Check sheet for the modelled part. Datum: model origin and axes. Units: mm. Coordinates: 2 decimals unless noted, no trailing zeros. Order: outer loops, then holes, each group sorted by start corner. A loop starts at its lowest first (then second) coordinate and runs counter-clockwise, first axis right, second up.
from build123d import *

# Parameters (mm, degrees)
EXTRUDE_1_DEPTH = 6
FILLET_1_R      = 0.5


with BuildPart() as part:
    # 草图1 → 凸台-拉伸1 (new body)
    with BuildSketch(Plane.XY):
        with BuildLine():
            Line((-9.3, 0), (-9.3, -15.9))
            Line((-9.3, -15.9), (9.3, -15.9))
            Line((9.3, -15.9), (9.3, 0))
            ThreePointArc((9.3, 0), (0, 9.3), (-9.3, 0))
        make_face()
    extrude(amount=EXTRUDE_1_DEPTH)

    # 圆角1
    fillet_1_edges = [part.edges().sort_by_distance(p)[0] for p in [
        (9.3, -15.9, 3),
        (-9.3, -15.9, 3),
    ]]
    fillet(fillet_1_edges, radius=FILLET_1_R)


solid = part.part
(1) Go/stop test with a flat-tipped pin: P1, Ø3, axis at x = 3, z = 2.5, coming from the +Y side. Record where the tip stops, or that it passes through.
Filled in:
P1: stops at y = 9.18
(2) Cross-section at A-A (z = 3.4). Enter the section's corners in (x, y).
Filled in:
outline: (-9.3, -15.4) arc R0.5 ccw to (-8.8, -15.9) - (8.8, -15.9) arc R0.5 ccw to (9.3, -15.4) - (9.3, 0) arc R9.3 ccw to (-9.3, 0) - close
(3) Thickness scan on probe 1 along Y at (x, z) = (7.5, 3.3); probe 2 along Y at (x, z) = (-3.75, 1.2); probe 3 along X at (y, z) = (2.25, 0.8). Record the ranges inside material, lowest first.
Filled in:
probe 1: y = -15.9 to 5.5
probe 2: y = -15.9 to 8.51
probe 3: x = -9.02 to 9.02
(4) Cross-section at B-B (x = 4.5). Enter the section's corners in (y, z), and give its area (3 significant figures).
Filled in:
outline: (-15.9, 0) - (8.14, 0) - (8.14, 6) - (-15.9, 6) - close
area: 144 mm2
(5) Cross-section at C-C (y = 4.5). Enter the section's corners in (x, z).
Filled in:
outline: (-8.14, 0) - (8.14, 0) - (8.14, 6) - (-8.14, 6) - close
